Could you check a few things on this model? Use its own coordinates, in mm. A direction names the side the tool comes from. Coordinates: 2 decimals unless noted, no trailing zeros. Loops run counter-clockwise (first coordinate to the right, second up) from the corner with the lowest first, then second, coordinate; pieces in that order, holes last. Notation, with made-up numbers: (0.25, 62.25) -> (5.25, 62.25) arc R23 ccw to (5.25, 83.25) -> close; hole circle Ø11 at (42.25, 18). An arc over 180 degrees is marked (long way). One line per question, with ' | ' between items. Start each with the question number.
(1) Suppose I cut it at D-D (z = 8.25). Please give me the cut outline in (x, y), plus the area to 3 significant figures.
(2) I'm going to push flat-ended pins straight in: pin 1 Ø3 at (x, z) = (-22, 6.5) entering from -Y; pin 2 Ø4 at (x, z) = (-35, 9) entering from -Y; pin 3 Ø2 at (x, z) = (8, 7) entering from -Y. Where does each tip first touch, or does it pass through?
(3) If I drill on line 1 along Y through (x, z) = (-16, 11.75); line 2 along Y through (x, z) = (10, 21); line 3 along X through (y, z) = (12.5, 4.25), over which ranges is the centre line in solid material (lowest first)?
(4) If we mould it in two halves opening along Y, with no side actions, what happens to faces 3 (the face through (-11.012, -49.592, 12.522)), 4 (the face through (16.733, 19.733, 12.522)), 5 (the face through (-1, 1, 25.4))? For each: pulls with the +Y half, pulls with the -Y half, needs draft (parallel to the pull), parting line crosses it, or undercut.
(5) Which directions (+Z, -Z, +X, -X, +Y, -Y) give clear straight access to the entire face, cutting with the end or side of a thin tool? Please do faces 1 (the face through (-1, 1, 0)), 2 (the face through (-6, -17.344, 13)).
(6) Suppose I cut it at B-B (y = 17.5). Please give me the cut outline in (x, z).
(7) Suppose I cut it at C-C (x = -15). Please give me the cut outline in (y, z).
(8) Suppose I cut it at A-A (x = 0). Please give me the cut outline in (y, z).
```python
from build123d import *

# Parameters (mm, degrees)
F0_R     = 50.8
F1_DEPTH = 25.4


with BuildPart() as f1:
    # F0 (on Top) → F1 (new body)
    with BuildSketch(Plane.XY):
        Circle(F0_R)
        Polygon((-3.934918, -40.953953), (-30.750657, -17.344443), (20.049343, -17.344443), align=None, mode=Mode.SUBTRACT)
        with BuildLine():
            ThreePointArc((-29.195861, -2.316432), (-20.606169, 19.678536), (-11.022453, -1.901868))
            ThreePointArc((-11.022453, -1.901868), (-20.181581, 1.065741), (-29.195861, -2.316432))
        make_face(mode=Mode.SUBTRACT)
        with BuildLine():
            ThreePointArc((10.762538, -0.96585), (17.137034, 19.739171), (23.408223, -0.997373))
            ThreePointArc((23.408223, -0.997373), (17.08885, 0.410144), (10.762538, -0.96585))
        make_face(mode=Mode.SUBTRACT)
    extrude(amount=F1_DEPTH)


solid = f1.part
```
Checks:
1) outline: circle Ø101.6 at (0, 0); hole (-30.75, -17.34) -> (-3.93, -40.95) -> (20.05, -17.34) -> close; hole (-29.2, -2.32) arc R14.59 cw to (-11.02, -1.9) arc R12.79 ccw (long way) to start; hole (10.76, -0.97) arc R15.06 cw to (23.41, -1) arc R11.33 ccw (long way) to start | area: 6,710 mm^2
2) pin 1: stops at y = -46.48 | pin 2: stops at y = -38.62 | pin 3: stops at y = -50.32
3) line 1: y = -48.21 to -30.33, -17.34 to 0.55, 18.93 to 48.21 | line 2: y = -49.81 to -27.24, -17.34 to -0.4, 17.23 to 49.81 | line 3: x = -49.24 to -31.81, -8.82 to 6.55, 27.67 to 49.24
4) face 3: parting line crosses it | face 4: undercut | face 5: needs draft
5) face 1: -Z, +X, -X, +Y, -Y | face 2: +Z, -Z
6) outline: (-47.69, 0) -> (-27.46, 0) -> (-27.46, 25.4) -> (-47.69, 25.4) -> close; (-13.17, 0) -> (10.35, 0) -> (10.35, 25.4) -> (-13.17, 25.4) -> close; (23.87, 0) -> (47.69, 0) -> (47.69, 25.4) -> (23.87, 25.4) -> close
7) outline: (-48.53, 0) -> (-31.21, 0) -> (-31.21, 25.4) -> (-48.53, 25.4) -> close; (-17.34, 0) -> (0.24, 0) -> (0.24, 25.4) -> (-17.34, 25.4) -> close; (18.53, 0) -> (48.53, 0) -> (48.53, 25.4) -> (18.53, 25.4) -> close
8) outline: (-50.8, 0) -> (-37.08, 0) -> (-37.08, 25.4) -> (-50.8, 25.4) -> close; (-17.34, 0) -> (50.8, 0) -> (50.8, 25.4) -> (-17.34, 25.4) -> close
